Autodesk Inventor part; units mm, degrees
ref_plane "YZ Plane" through (0, 0, 0) normal (1, 0, 0) x (0, 1, 0)
ref_plane "XZ Plane" through (0, 0, 0) normal (0, 1, 0) x (-1, 0, 0)
ref_plane "XY Plane" through (0, 0, 0) normal (0, 0, 1) x (1, 0, 0)
sketch "Sketch1" plane through (0, 0, 0) normal (0, 0, 1) x (1, 0, 0)
  line L0 (0, 54.6) -> (0, -54.6) construction
  line L1 (-54.6, 0) -> (54.6, 0) construction
  line L2 (-39, 39) -> (39, 39)
  line L3 (39, 39) -> (39, -39)
  line L4 (39, -39) -> (-39, -39)
  line L5 (-39, -39) -> (-39, 39)
  point P0 (0, 0)
  dimension "d0" = 78
  dimension "d1" = 78
extrude "Extrusion1" add sketch "Sketch1" along normal blind 80
sketch "Sketch2" plane through (0, 0, 0) normal (0, 0, -1) x (-1, 0, 0)
  circle A0 centre (0, 0) radius 27.5
  circle A1 centre (0, 0) radius 23.5
  dimension "d4" = 55
  dimension "d5" = 47
extrude "Extrusion2" add sketch "Sketch2" along normal blind 38
properties part number "Iris15_Volume_Incorrect"
Part model, mm, in its own coordinate system. A direction names the side the tool comes from. Round coordinates to 2 decimals unless told otherwise and drop trailing zeros. Order: outer loops, then holes, each group sorted by start corner. A loop starts at its lowest first (then second) coordinate and runs counter-clockwise, first axis right, second up. Notation, with made-up numbers: M -36.75,-19.75 L -3.75,-19.75 A19 ccw -3.75,-9.75 Z; hole C 54.25,-32 d7. An arc over 180 degrees is marked long. Put each result on its own line as item: value. Start each with the question number.
1. Drop flat-ended pins along their axis: pin 1 (1 mm diameter, centred on x = -1, y = -18, fed in from -Z); pin 2 (6 mm diameter, centred on x = -6, z = -16.5, fed in from +Y). Give the stop position or say it passes through.
2. Slice it at A-A on x = 0. List the corners of the cut face in (y, z), then the cut area to 3 significant figures.
3. Slice it at D-D on x = -26. List the corners of the cut face in (y, z), then the cut area to 3 significant figures.
4. Drill centre lines: probe 1 along Y at (x, z) = (0, -20.5); probe 2 along Z at (x, y) = (21, 3.5); probe 3 along X at (y, z) = (8, -5.5). Where is each one in solid material? Low to high. Write a range as [from, to].
5. Tool access for faces 4 (the face through (5.961, 26.846, -18.734)), 5 (the face through (-1, 39, 39)): list every direction of +Z, -Z, +X, -X, +Y, -Y with a clear straight run to the whole face (end or side of a thin tool).
6. Slice it at C-C on z = -29. List the corners of the cut face in (x, y), then the cut area to 3 significant figures.
7. Two-plate mould, pull along X, no slides. Class faces 1 (the face through (39, 1, 39)), 2 (the face through (-9, 27, 0)), 3 (the face through (0, 0, 0)): +X half, -X half, draft (parallel to the pull), parting line (faces both ways), or undercut.
Findings:
1. pin 1: z = 0
1. pin 2: y = 27.34
2. outline: M -39,0 L -27.5,0 L -27.5,-38 L -23.5,-38 L -23.5,0 L 23.5,0 L 23.5,-38 L 27.5,-38 L 27.5,0 L 39,0 L 39,80 L -39,80 Z
2. area: 6,540 mm2
3. outline: M -39,0 L -8.96,0 L -8.96,-38 L 8.96,-38 L 8.96,0 L 39,0 L 39,80 L -39,80 Z
3. area: 6,920 mm2
4. probe 1: [-27.5, -23.5], [23.5, 27.5]
4. probe 2: [0, 80]
4. probe 3: [-26.31, -22.1], [22.1, 26.31]
5. face 4: -Z
5. face 5: +Z, -Z, +X, -X, +Y
6. outline: C 0,0 d55; hole C 0,0 d47
6. area: 641 mm2
7. face 1: +X half
7. face 2: draft
7. face 3: undercut
